from build123d import *

# Parameters (mm, degrees)
F0_W     = 600
F0_H     = 600
F1_DEPTH = 40
F2_W     = 55.912304
F2_H     = 55.912304
F3_DEPTH = 400
F5_W     = 600
F5_H     = 600
F6_DEPTH = 40
F7_R     = 20


with BuildPart() as f1:
    # F0 (on Top) → F1 (new body)
    with BuildSketch(Plane.XY):
        Rectangle(F0_W, F0_H)
    extrude(amount=F1_DEPTH)

    # F2 (on face) → F3 (join)
    with BuildSketch(Plane(origin=(0, 0, 0), x_dir=(1, 0, 0), z_dir=(0, 0, -1))):
        with Locations((-272.043848, 272.043848)):
            Rectangle(F2_W, F2_H)
        with Locations((272.043848, 272.043848)):
            Rectangle(F2_W, F2_H)
        with Locations((272.043848, -272.043848)):
            Rectangle(F2_W, F2_H)
        with Locations((-272.043848, -272.043848)):
            Rectangle(F2_W, F2_H)
    extrude(amount=F3_DEPTH)

    # F5 (on offset) → F6 (join)
    with BuildSketch(Plane.XY.offset(-280)):
        Rectangle(F5_W, F5_H)
    extrude(amount=-F6_DEPTH)

    # F7
    f7_edges = [f1.edges().sort_by_distance(p)[0] for p in [
        (300, -300, -180),
        (-300, -300, -180),
        (300, 300, -180),
        (-300, 300, -180),
    ]]
    fillet(f7_edges, radius=F7_R)


solid = f1.part
The model under review builds one solid part; all positions refer to its coordinate system, in mm. A direction names the side the tool comes from. Coordinates: 2 decimals unless noted, no trailing zeros. Write each loop counter-clockwise with the first axis right and the second up, starting at its lowest first coordinate (ties: lowest second). Pieces come first, ordered by that corner, then holes. Notation, with made-up numbers: (35, 68) -> (56, 68) arc R25 ccw to (56, 100) -> close; hole circle Ø3 at (59, 55). An arc over 180 degrees is marked (long way). Answer in a Markdown table with one row per item.
1. Draft analysis for pull direction Z (two halves, no side actions). For faces 1 (the flat face through (272, -244.088, -138)), 2 (the flat face through (272, 272, -400)), 3 (the flat face through (-1, -300, -309)), state which applies: +Z half, -Z half, draft (parallel to the pull), parting line (faces both ways), or undercut.
Answers below:
| item | result |
|---|---|
| face 1 | undercut |
| face 2 | -Z half |
| face 3 | draft |
2. We need section D-D, the plane x = -263. State the section outline as (y, z) points, and give its area (3 significant figures).
Answers below:
| item | result |
|---|---|
| outline | (-300, -400) -> (-244.09, -400) -> (-244.09, -320) -> (244.09, -320) -> (244.09, -400) -> (300, -400) -> (300, 40) -> (-300, 40) -> close; hole (-244.09, -280) -> (244.09, -280) -> (244.09, 0) -> (-244.09, 0) -> close |
| area | 88,300 mm^2 |
3. For faces 4 (the flat face through (-4, 4, 0)), 5 (the flat face through (-244.088, 272, -138)), 6 (the flat face through (-272, 244.088, -359)), 7 (the flat face through (-244.088, 272, -359)), 8 (the flat face through (-272, 244.088, -138)), list the 3-axis set-ups (+Z, -Z, +X, -X, +Y, -Y) from which the entire face can be reached by the end or side of a thin tool; tool diameter is ignored.
Answers below:
| item | result |
|---|---|
| face 4 | none |
| face 5 | +Y, -Y |
| face 6 | -Z, +X, -X |
| face 7 | -Z, +Y, -Y |
| face 8 | +X, -X |
4. We need section A-A, the plane z = -144. State the section outline as (x, y) points, and give its area (3 significant figures).
Answers below:
| item | result |
|---|---|
| outline | (-300, -280) arc R20 ccw to (-280, -300) -> (-244.09, -300) -> (-244.09, -244.09) -> (-300, -244.09) -> close; (-300, 244.09) -> (-244.09, 244.09) -> (-244.09, 300) -> (-280, 300) arc R20 ccw to (-300, 280) -> close; (244.09, -300) -> (280, -300) arc R20 ccw to (300, -280) -> (300, -244.09) -> (244.09, -244.09) -> close; (244.09, 244.09) -> (300, 244.09) -> (300, 280) arc R20 ccw to (280, 300) -> (244.09, 300) -> close |
| area | 12,200 mm^2 |
5. We need section B-B, the plane x = 22. State the section outline as (y, z) points, and give its area (3 significant figures).
Answers below:
| item | result |
|---|---|
| outline | (-300, -320) -> (300, -320) -> (300, -280) -> (-300, -280) -> close; (-300, 0) -> (300, 0) -> (300, 40) -> (-300, 40) -> close |
| area | 48,000 mm^2 |
6. Wall thickness on probe 1 along Z at (x, y) = (-98, -54); probe 2 along Y at (x, z) = (258.5, -364): over which ranges is each line inside the solid? List them lowest first. Write a range as [from, to].
Answers below:
| item | result |
|---|---|
| probe 1 | z = [-320, -280], [0, 40] |
| probe 2 | y = [-300, -244.09], [244.09, 300] |
